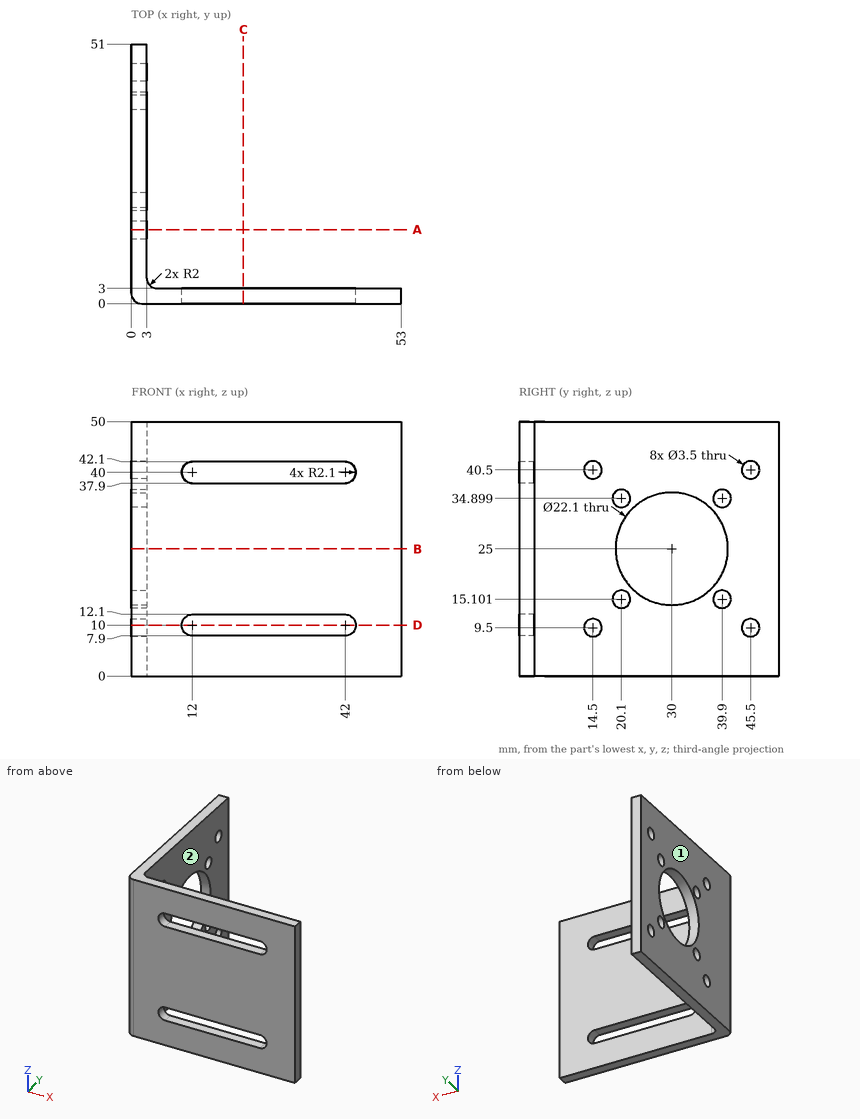
Part print with two shaded views. Sizes in mm from the minimum x, y, z corner. A direction names the side the tool comes from. Coordinates: 2 decimals unless noted, no trailing zeros. Write each loop counter-clockwise with the first axis right and the second up, starting at its lowest first coordinate (ties: lowest second). Pieces come first, ordered by that corner, then holes. Notation, with made-up numbers: (39, 2.25) - (53, 2.25) arc R29 ccw to (53, 40.25) - close; hole circle Ø2 at (-25, 32). An arc over 180 degrees is marked (long way). One line per item, written item: value. Start each with the question number.
1. Slice it at B-B (z = 25). Write the cut outline in (x, y).
2. Slice it at C-C (x = 22). Write the cut outline in (y, z).
3. Probe line 1 (Z direction, x = 2, y = 20); line 2 (X direction, y = 10.5, z = 31). List the from-to ranges inside material, lowest first. Write a range as from..to.
4. Slice it at D-D (z = 10). Write the cut outline in (x, y), plus the area to 3 significant figures.
5. Tool access for the marked faces 1 and 2: list every direction of +Z, -Z, +X, -X, +Y, -Y with a clear straight run to the whole face (end or side of a thin tool).
6. Flat gauge pins, fed straight in: pin 1 (5.5 mm diameter, centred on y = 20.1, z = 34.9, fed in from +X); pin 2 (10 mm diameter, centred on x = 26.5, z = 29, fed in from +Y); pin 3 (6 mm diameter, centred on y = 31.5, z = 32.5, fed in from -X) (1 decimal). Where does each tip first touch, or does it go through?
7. Slice it at A-A (y = 14.5). Write the cut outline in (x, z).
Answers below:
1. outline: (0, 2) arc R2 ccw to (2, 0) - (53, 0) - (53, 3) - (5, 3) arc R2 cw to (3, 5) - (3, 18.95) - (0, 18.95) - close; (0, 41.05) - (3, 41.05) - (3, 51) - (0, 51) - close
2. outline: (0, 0) - (3, 0) - (3, 7.9) - (0, 7.9) - close; (0, 12.1) - (3, 12.1) - (3, 37.9) - (0, 37.9) - close; (0, 42.1) - (3, 42.1) - (3, 50) - (0, 50) - close
3. line 1: z = 0..13.35, 16.85..20.3, 29.7..33.15, 36.65..50
3. line 2: x = 0..3
4. outline: (0, 2) arc R2 ccw to (2, 0) - (9.9, 0) - (9.9, 3) - (5, 3) arc R2 cw to (3, 5) - (3, 12.82) - (0, 12.82) - close; (0, 16.18) - (3, 16.18) - (3, 43.82) - (0, 43.82) - close; (0, 47.18) - (3, 47.18) - (3, 51) - (0, 51) - close; (44.1, 0) - (53, 0) - (53, 3) - (44.1, 3) - close
4. area: 180 mm^2
5. face 1: +Z, -Z, -X, +Y, -Y
5. face 2: +Z, -Z, +X, +Y
6. pin 1: stops at x = 3
6. pin 2: stops at y = 3
6. pin 3: passes through
7. outline: (0, 0) - (3, 0) - (3, 7.75) - (0, 7.75) - close; (0, 11.25) - (3, 11.25) - (3, 38.75) - (0, 38.75) - close; (0, 42.25) - (3, 42.25) - (3, 50) - (0, 50) - close
